Geometry: final body of the model. Coordinates: model frame, mm. Face numbers are marked on the shaded views. Give positions to 0.01 mm unless a question says otherwise; leave off trailing zeros. Write each loop counter-clockwise with the first axis right and the second up, starting at its lowest first coordinate (ties: lowest second). Pieces come first, ordered by that corner, then holes. Notation, with made-up numbers: M 65.25,74 L 69.25,74 A8 ccw 69.25,80 Z; hole C 74.25,37.5 d4. An arc over 180 degrees is marked long. Use one line per item in the form item = value. Start each with the question number.
Item 1: Section query D-D on y = 2.75. Return loops of the section in (x, z).
Item 2: Material intervals for line 1 along Y through (x, z) = (29, 3.2); line 2 along X through (y, z) = (15.5, 1); line 3 along X through (y, z) = (4.5, 1.25), sorted ascending. Write a range as from..to.
Item 3: Pull-direction query (X, two-part tool) for the marked faces 1, 2 and 3; classes: released by +X, released by -X, zero draft, split by the parting line, or undercut.
Item 4: Section query C-C on x = 17.5. Return loops of the section in (y, z).
Item 5: Section query B-B on y = 12.75. Return loops of the section in (x, z).
Item 6: Section query A-A on x = 11. Return loops of the section in (y, z), then the cut area to 3 significant figures.
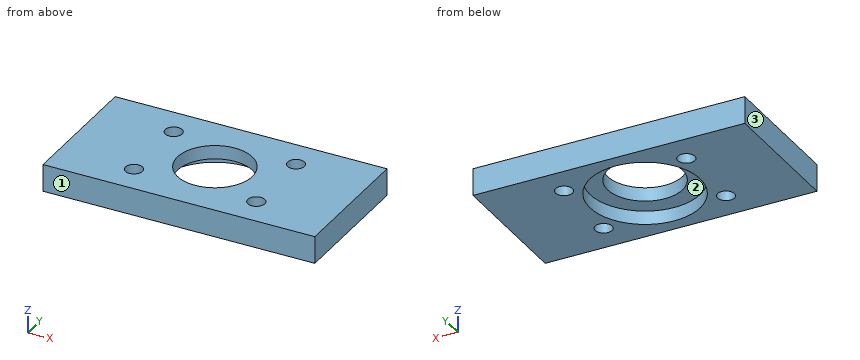
Autodesk Inventor part; units mm, degrees
ref_plane "YZ Plane" through (0, 0, 0) normal (1, 0, 0) x (0, 1, 0)
ref_plane "XZ Plane" through (0, 0, 0) normal (0, 1, 0) x (-1, 0, 0)
ref_plane "XY Plane" through (0, 0, 0) normal (0, 0, 1) x (1, 0, 0)
sketch "Sketch1" plane through (0, 0, 0) normal (0, 0, 1) x (1, 0, 0)
  line L0 (0, 0) -> (40, 0)
  line L1 (40, 0) -> (40, 20)
  line L2 (40, 20) -> (0, 20)
  line L3 (0, 20) -> (0, 0)
  dimension "d0" = 40
  dimension "d1" = 20
extrude "Extrusion1" add sketch "Sketch1" along normal blind 4
sketch "Sketch3" plane through (0, 0, 4) normal (0, 0, 1) x (1, 0, 0)
  line L0 (40, 20) -> (0, 20)
  line L1 (0, 20) -> (0, 0)
  point P0 (11, 15.5)
  dimension "d41" = 4.5
  dimension "d42" = 11
hole "Hole2" at (11, 15.5, 4) direction (0, 0, -1) diameter 2.5 end through all
sketch "Sketch4" plane through (0, 0, 4) normal (0, 0, 1) x (1, 0, 0)
  line L0 (0, 20) -> (0, 0)
  line L1 (0, 0) -> (40, 0)
  point P0 (11, 4.5)
  dimension "d43" = 11
  dimension "d44" = 4.5
hole "Hole3" at (11, 4.5, 4) direction (0, 0, -1) diameter 2.5 end through all
sketch "Sketch5" plane through (0, 0, 4) normal (0, 0, 1) x (1, 0, 0)
  line L0 (40, 0) -> (40, 20)
  line L1 (40, 20) -> (0, 20)
  point P0 (0, 0)
  point P1 (29, 15.5)
  dimension "d45" = 11
  dimension "d46" = 4.5
hole "Hole4" at (29, 15.5, 4) direction (0, 0, -1) diameter 2.5 end through all
sketch "Sketch6" plane through (0, 0, 4) normal (0, 0, 1) x (1, 0, 0)
  line L0 (40, 0) -> (40, 20)
  line L1 (0, 0) -> (40, 0)
  point P0 (29, 4.5)
  dimension "d47" = 11
  dimension "d48" = 4.5
hole "Hole5" at (29, 4.5, 4) direction (0, 0, -1) diameter 2.5 end through all
sketch "Sketch7" plane through (0, 0, 0) normal (0, 0, -1) x (-1, 0, 0)
  line L0 (0, 20) -> (0, 0)
  line L1 (-40, 20) -> (0, 20)
  point P0 (-19.9898, 9.9924)
  dimension "d56" = 19.9898
  dimension "d57" = 10.0076
hole "Hole6" at (19.9898, 9.9924, 0) direction (0, 0, 1) diameter 11 end through all counterbore diameter 16.2 counterbore depth 2
properties part number "bottom_g2v1"
Answer sheet:
q1.outline = M 0,0 L 16.36,0 L 16.36,2 L 23.62,2 L 23.62,0 L 40,0 L 40,4 L 0,4 Z
q2.line_1 = 0..3.25, 5.75..14.25, 16.75..20
q2.line_2 = 0..9.75, 12.25..14.05, 25.93..27.75, 30.25..40
q2.line_3 = 0..9.75, 12.25..14.04, 25.94..27.75, 30.25..40
q3.face_1 = zero draft
q3.face_2 = undercut
q3.face_3 = released by -X
q4.outline = M 0,0 L 2.28,0 L 2.28,2 L 5.09,2 L 5.09,4 L 0,4 Z; M 14.9,2 L 17.7,2 L 17.7,0 L 20,0 L 20,4 L 14.9,4 Z
q5.outline = M 0,0 L 12.37,0 L 12.37,2 L 15.23,2 L 15.23,4 L 0,4 Z; M 24.75,2 L 27.61,2 L 27.61,0 L 40,0 L 40,4 L 24.75,4 Z
q6.outline = M 0,0 L 3.25,0 L 3.25,4 L 0,4 Z; M 5.75,0 L 14.25,0 L 14.25,4 L 5.75,4 Z; M 16.75,0 L 20,0 L 20,4 L 16.75,4 Z
q6.area = 60.0 mm2
